The model under review builds one solid part; all positions refer to its coordinate system, in mm. Face numbers are marked on the shaded views. Give positions to 0.01 mm unless a question says otherwise; leave off trailing zeros. Order: outer loops, then holes, each group sorted by start corner. A loop starts at its lowest first (then second) coordinate and runs counter-clockwise, first axis right, second up.
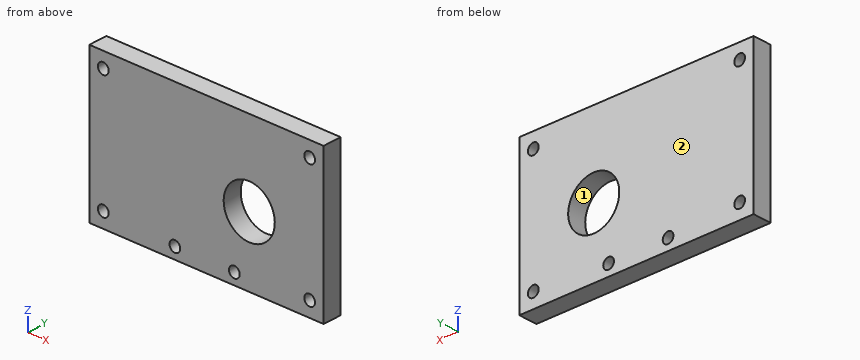
```python
from build123d import *

# Parameters (mm, degrees)
SKETCH1_W           = 80.01
SKETCH1_H           = 50.8
BOSS_EXTRUDE1_DEPTH = 6.35
SKETCH2_R           = 1.8415
CUT_EXTRUDE1_DEPTH  = 48.81090383
SKETCH3_R           = 8.73125
SKETCH3_R_2         = 1.8288
CUT_EXTRUDE2_DEPTH  = 48.81090383


with BuildPart() as part:
    # Sketch1 → Boss-Extrude1 (new body)
    with BuildSketch(Plane(origin=(0, 0, 0), x_dir=(1, 0, 0), z_dir=(0, 1, 0))):
        Rectangle(SKETCH1_W, SKETCH1_H)
    extrude(amount=BOSS_EXTRUDE1_DEPTH)

    # Sketch2 → Cut-Extrude1 (cut, through all)
    with BuildSketch(Plane(origin=(0, 6.35, 0), x_dir=(1, 0, 0), z_dir=(0, 1, 0))):
        with Locations(Location((-35.2425, 20.32, 0), (0, 0, 270))):
            Circle(SKETCH2_R)
        with Locations(Location((-35.2425, -20.32, 0), (0, 0, 270))):
            Circle(SKETCH2_R)
        with Locations(Location((35.2425, -20.32, 0), (0, 0, 270))):
            Circle(SKETCH2_R)
        with Locations(Location((35.2425, 20.32, 0), (0, 0, 270))):
            Circle(SKETCH2_R)
    extrude(amount=-CUT_EXTRUDE1_DEPTH, mode=Mode.SUBTRACT)

    # Sketch3 → Cut-Extrude2 (cut, through all)
    with BuildSketch(Plane(origin=(0, 6.35, 0), x_dir=(1, 0, 0), z_dir=(0, 1, 0))):
        with Locations(Location((14.605, 2.54, 0), (0, 0, 270))):
            Circle(SKETCH3_R)
        with Locations(Location((-10.795, 21.59, 0), (0, 0, 270))):
            Circle(SKETCH3_R_2)
        with Locations(Location((9.525, 21.59, 0), (0, 0, 270))):
            Circle(SKETCH3_R_2)
    extrude(amount=-CUT_EXTRUDE2_DEPTH, mode=Mode.SUBTRACT)


solid = part.part
```
Item 1: Take a section at C-C (x = 13.5). Give the boundary of the cut face in (y, z), and give its area (3 significant figures).
Values found:
outline: (0, -25.4) - (6.35, -25.4) - (6.35, -11.2) - (0, -11.2) - close; (0, 6.12) - (6.35, 6.12) - (6.35, 25.4) - (0, 25.4) - close
area: 213 mm2
Item 2: Draft analysis for pull direction Z (two halves, no side actions). For the marked faces 1 and 2, state which applies: released by +Z, released by -Z, zero draft, split by the parting line, or undercut.
Values found:
face 1: undercut
face 2: zero draft
Item 3: Take a section at B-B (z = -2.54). Give the boundary of the cut face in (x, y) (3 decimals).
Values found:
outline: (-40.005, 0) - (5.874, 0) - (5.874, 6.35) - (-40.005, 6.35) - close; (23.336, 0) - (40.005, 0) - (40.005, 6.35) - (23.336, 6.35) - close
Item 4: For line 1 (X direction, y = 2.25, z = 20.32) (3 decimals); line 2 (X direction, y = 1.5, z = -2) (3 decimals); line 3 (X direction, y = 5, z = -21.59) (3 decimals), list the stretches that pass through material, from the lowest coordinate up.
Values found:
line 1: x = -40.005 to -37.084, -33.401 to 33.401, 37.084 to 40.005
line 2: x = -40.005 to 5.89, 23.32 to 40.005
line 3: x = -40.005 to -36.576, -33.909 to -12.624, -8.966 to 7.696, 11.354 to 33.909, 36.576 to 40.005
Item 5: Take a section at D-D (y = 4). Give the boundary of the cut face in (x, z) (1 decimal), and give its area (3 significant figures).
Values found:
outline: (-40, -25.4) - (40, -25.4) - (40, 25.4) - (-40, 25.4) - close; hole circle Ø3.7 at (-35.2, -20.3); hole circle Ø3.7 at (-35.2, 20.3); hole circle Ø3.7 at (-10.8, -21.6); hole circle Ø17.5 at (14.6, -2.5); hole circle Ø3.7 at (9.5, -21.6); hole circle Ø3.7 at (35.2, -20.3); hole circle Ø3.7 at (35.2, 20.3)
area: 3,760 mm2
Item 6: Take a section at A-A (z = 20.32). Give the boundary of the cut face in (x, y) (3 decimals), and give its area (3 significant figures).
Values found:
outline: (-40.005, 0) - (-37.084, 0) - (-37.084, 6.35) - (-40.005, 6.35) - close; (-33.401, 0) - (33.401, 0) - (33.401, 6.35) - (-33.401, 6.35) - close; (37.084, 0) - (40.005, 0) - (40.005, 6.35) - (37.084, 6.35) - close
area: 461 mm2
Item 7: Clearance check with flat-ended pins moving along their axes: pin 1 Ø4 at (x, z) = (9.525, -21.59) entering from -Y; pin 2 Ø10.5 at (x, z) = (14.605, -2.54) entering from -Y (3 decimals). State where each tip first meets the part, or that it passes through.
Values found:
pin 1: stops at y = 0
pin 2: passes through
